from build123d import *

# Parameters (mm, degrees)
SKETCH_1_R          = 2.75
EXTRUDE_1_DEPTH     = 3
FILLET_1_R          = 0.5
CUT_EXTRUDE_1_DEPTH = 2
SKETCH_3_R          = 1.5
EXTRUDE_2_DEPTH     = 14
CHAMFER_1_SIZE      = 0.2
FILLET_2_R          = 0.2


with BuildPart() as part:
    # 草图1 → 凸台-拉伸1 (new body)
    with BuildSketch(Plane.XY):
        Circle(SKETCH_1_R)
    extrude(amount=EXTRUDE_1_DEPTH)

    # 圆角1
    fillet_1_edges = [part.edges().sort_by_distance(p)[0] for p in [
        (-2.75, 0, 3),
    ]]
    fillet(fillet_1_edges, radius=FILLET_1_R)

    # 草图2 → 切除-拉伸1 (cut)
    with BuildSketch(Plane.XY.offset(3)):
        Polygon((1.558845727, 0), (0.779422863, 1.35), (-0.779422863, 1.35), (-1.558845727, 0), (-0.779422863, -1.35), (0.779422863, -1.35), align=None)
    extrude(amount=-CUT_EXTRUDE_1_DEPTH, mode=Mode.SUBTRACT)

    # 草图3 → 凸台-拉伸2 (add)
    with BuildSketch(Plane(origin=(0, 0, 0), x_dir=(-1, 0, 0), z_dir=(0, 0, -1))):
        Circle(SKETCH_3_R)
    extrude(amount=EXTRUDE_2_DEPTH)

    # 倒角1
    chamfer_1_edges = [part.edges().sort_by_distance(p)[0] for p in [
        (1.5, 0, -14),
    ]]
    chamfer(chamfer_1_edges, length=CHAMFER_1_SIZE)

    # 圆角2
    fillet_2_edges = [part.edges().sort_by_distance(p)[0] for p in [
        (-2.75, 0, 0),
    ]]
    fillet(fillet_2_edges, radius=FILLET_2_R)


solid = part.part
Can you work these out from the model? Positions are in its coordinate system, mm. A direction names the side the tool comes from. Round coordinates to 2 decimals unless told otherwise and drop trailing zeros. Loops run counter-clockwise (first coordinate to the right, second up) from the corner with the lowest first, then second, coordinate; pieces in that order, holes last. Notation, with made-up numbers: (-22, 73.5) - (-10, 73.5) arc R12 cw to (-10, 80.5) - close; hole circle Ø11 at (67, -1). An arc over 180 degrees is marked (long way). Use CSV: the item, a comma, the result in double quotes. Start each with the question number.
1) For pin 1 Ø1.5 at (x, z) = (-1, -2.5) entering from -Y; pin 2 Ø2 at (y, z) = (-1.5, -1.5) entering from +X, each with a flat end and sliding along its axis, tell me the tip position at first contact or that it passes through.
2) If we section it at B-B on x = 0: Write out the boundary of the cut face in (y, z).
3) If we section it at A-A on z = 1.25: Write out the boundary of the cut face in (x, y), plus the area to 3 significant figures.
4) Please list where these lines run through material, in increasing order: probe 1 along Z at (x, y) = (-0.7, -0.85); probe 2 along Z at (x, y) = (0, -2.2); probe 3 along X at (y, z) = (0.2, -5.5). Write a range as [from, to].
5) If we section it at C-C on z = -9.25: Write out the boundary of the cut face in (x, y), plus the area to 3 significant figures.
6) We'd pull the mould along Y, two halves only. Please class faces 4 (the flat face through (0, -1.35, 2)), 5 (the cylindrical face through (-0.596, -2.685, 1.334)), 6 (the flat face through (0, 0, -14)), 7 (the flat face through (1.17, 0.67, 2.01)): released by +Y, released by -Y, zero draft, split by the parting line, or undercut.
7) For faces 1 (the flat face through (1.5, -0.5, 3)), 2 (the flat face through (1.164, -0.684, 2.014)), 3 (the cylindrical face through (1.5, 0.07, -6.8)), which set-ups out of +Z, -Z, +X, -X, +Y, -Y let a thin tool reach every point of the face, with its end or its side?
Geometry results:
1,pin 1,"stops at y = -1.48"
1,pin 2,"stops at x = 1.41"
2,outline,"(-2.75, 0.2) arc R0.2 ccw to (-2.55, 0) - (-1.5, 0) - (-1.5, -13.8) - (-1.3, -14) - (1.3, -14) - (1.5, -13.8) - (1.5, 0) - (2.55, 0) arc R0.2 ccw to (2.75, 0.2) - (2.75, 2.5) arc R0.5 ccw to (2.25, 3) - (1.35, 3) - (1.35, 1) - (-1.35, 1) - (-1.35, 3) - (-2.25, 3) arc R0.5 ccw to (-2.75, 2.5) - close"
3,outline,"circle Ø5.5 at (0, 0); hole (-1.56, 0) - (-0.78, -1.35) - (0.78, -1.35) - (1.56, 0) - (0.78, 1.35) - (-0.78, 1.35) - close"
3,area,"17.4 mm2"
4,probe 1,"z = [-14, 1]"
4,probe 2,"z = [0, 3]"
4,probe 3,"x = [-1.49, 1.49]"
5,outline,"circle Ø3 at (0, 0)"
5,area,"7.07 mm2"
6,face 4,"undercut"
6,face 5,"split by the parting line"
6,face 6,"zero draft"
6,face 7,"undercut"
7,face 1,"+Z, +X, -X, +Y, -Y"
7,face 2,"+Z"
7,face 3,"-Z"
